Part model, mm, in its own coordinate system. A direction names the side the tool comes from. Give positions to 0.01 mm unless a question says otherwise; leave off trailing zeros. Order: outer loops, then holes, each group sorted by start corner. A loop starts at its lowest first (then second) coordinate and runs counter-clockwise, first axis right, second up.
1. Drop flat-ended pins along their axis: pin 1 Ø0.8 at (y, z) = (3, 2) entering from +X; pin 2 Ø1 at (x, y) = (11, 2) entering from +Z; pin 3 Ø4 at (x, z) = (5, 12.5) entering from -Y; pin 4 Ø1.5 at (x, y) = (5, -4.5) entering from +Z. Give the stop position or say it passes through.
2. Which spindle directions (+Z, -Z, +X, -X, +Y, -Y) get a long thin tool onto all of the face, cutting with end or side? Do faces 1 (the flat face through (14, -1, 3.345)), 2 (the flat face through (14, 1.4, 25)), 3 (the flat face through (22.64, -1, 2)). Say none if no direction does.
3. Mould opens along X. For faces 4 (the flat face through (14, 1, 27.5)), 5 (the flat face through (4.86, -1, 2)), 6 (the flat face through (14, -2.54, 3)), 7 (the cylindrical face through (26.84, 0.69, 1.72)) say: +X half, -X half, draft (parallel to the pull), parting line (faces both ways), or undercut.
4. Probe line 1 (X direction, y = 0.7, z = 1.9); line 2 (Y direction, x = 24.75, z = 16); line 3 (Y direction, x = 17.75, z = 4). List the from-to ranges inside material, lowest first.
5. Slice it at C-C on y = -5.5. List the corners of the cut face in (x, z) (3 decimals), and give its area (3 significant figures).
6. Slice it at B-B on z = 25.6. List the corners of the cut face in (x, y), and give its area (3 significant figures).
7. Slice it at D-D on y = 0.75. List the corners of the cut face in (x, z), and give its area (3 significant figures).
8. Slice it at A-A on x = 2.05. List the corners of the cut face in (y, z), and give its area (3 significant figures).
from build123d import *

# Parameters (mm, degrees)
SKETCH_1_W      = 27.5
SKETCH_1_H      = 27.5
SKETCH_1_R      = 1.4
EXTRUDE_1_DEPTH = 1.4
SKETCH_1_3_W    = 27.5
SKETCH_1_3_H    = 19.2
EXTRUDE_2_DEPTH = 3
SKETCH_1_4_W    = 2.54
SKETCH_1_4_H    = 2.54
EXTRUDE_3_DEPTH = 2.54
EXTRUDE_START   = 3.4
SKETCH_1_5_W    = 0.7
SKETCH_1_5_H    = 0.7
EXTRUDE_4_DEPTH = 11.3


with BuildPart() as part:
    # Sketch 1 → Extrude 1 (new body)
    with BuildSketch(Plane(origin=(0, 0, 0), x_dir=(1, 0, 0), z_dir=(0, 1, 0))):
        with Locations((13.75, -13.75)):
            Rectangle(SKETCH_1_W, SKETCH_1_H)
        with Locations(Location((2.05, -1.9, 0), (0, 0, 270))):
            Circle(SKETCH_1_R, mode=Mode.SUBTRACT)
        with Locations(Location((25.45, -1.9, 0), (0, 0, 270))):
            Circle(SKETCH_1_R, mode=Mode.SUBTRACT)
        with Locations(Location((2.05, -25.6, 0), (0, 0, 270))):
            Circle(SKETCH_1_R, mode=Mode.SUBTRACT)
        with Locations(Location((25.45, -25.6, 0), (0, 0, 270))):
            Circle(SKETCH_1_R, mode=Mode.SUBTRACT)
    extrude(amount=EXTRUDE_1_DEPTH)

    # Sketch 1_3 → Extrude 2 (add)
    with BuildSketch(Plane(origin=(0, 0, 0), x_dir=(1, 0, 0), z_dir=(0, 1, 0))):
        with Locations((13.75, -13.75)):
            Rectangle(SKETCH_1_3_W, SKETCH_1_3_H)
    extrude(amount=EXTRUDE_2_DEPTH)

    # Sketch 1_4 → Extrude 3 (add)
    with BuildSketch(Plane(origin=(0, 0, 0), x_dir=(1, 0, 0), z_dir=(0, 1, 0))):
        with Locations((6.13, -2.075)):
            Rectangle(SKETCH_1_4_W, SKETCH_1_4_H)
        with Locations((8.67, -2.075)):
            Rectangle(SKETCH_1_4_W, SKETCH_1_4_H)
        with Locations((11.21, -2.075)):
            Rectangle(SKETCH_1_4_W, SKETCH_1_4_H)
        with Locations((13.75, -2.075)):
            Rectangle(SKETCH_1_4_W, SKETCH_1_4_H)
        with Locations((16.29, -2.075)):
            Rectangle(SKETCH_1_4_W, SKETCH_1_4_H)
        with Locations((18.83, -2.075)):
            Rectangle(SKETCH_1_4_W, SKETCH_1_4_H)
        with Locations((21.37, -2.075)):
            Rectangle(SKETCH_1_4_W, SKETCH_1_4_H)
    extrude(amount=-EXTRUDE_3_DEPTH)

    # Sketch 1_5 → Extrude 4 (add)
    with BuildSketch(Plane(origin=(0, 0, 0), x_dir=(1, 0, 0), z_dir=(0, 1, 0)).offset(EXTRUDE_START)):
        with Locations((6.13, -2.075)):
            Rectangle(SKETCH_1_5_W, SKETCH_1_5_H)
        with Locations((8.67, -2.075)):
            Rectangle(SKETCH_1_5_W, SKETCH_1_5_H)
        with Locations((11.21, -2.075)):
            Rectangle(SKETCH_1_5_W, SKETCH_1_5_H)
        with Locations((13.75, -2.075)):
            Rectangle(SKETCH_1_5_W, SKETCH_1_5_H)
        with Locations((16.29, -2.075)):
            Rectangle(SKETCH_1_5_W, SKETCH_1_5_H)
        with Locations((18.83, -2.075)):
            Rectangle(SKETCH_1_5_W, SKETCH_1_5_H)
        with Locations((21.37, -2.075)):
            Rectangle(SKETCH_1_5_W, SKETCH_1_5_H)
    extrude(amount=-EXTRUDE_4_DEPTH)


solid = part.part
Data:
1. pin 1: stops at x = 21.72
1. pin 2: stops at z = 23.35
1. pin 3: stops at y = 0
1. pin 4: passes through
2. face 1: +Z, +X, -X, -Y
2. face 2: +Z, +X, -X, +Y
2. face 3: +Z, -Z, +X, -Y
3. face 4: draft
3. face 5: -X half
3. face 6: undercut
3. face 7: undercut
4. line 1: x = 0 to 0.65, 3.45 to 24.05, 26.85 to 27.5
4. line 2: y = 0 to 3
4. line 3: y = 0 to 1.4
5. outline: (5.78, 1.725) - (6.48, 1.725) - (6.48, 2.425) - (5.78, 2.425) - close; (8.32, 1.725) - (9.02, 1.725) - (9.02, 2.425) - (8.32, 2.425) - close; (10.86, 1.725) - (11.56, 1.725) - (11.56, 2.425) - (10.86, 2.425) - close; (13.4, 1.725) - (14.1, 1.725) - (14.1, 2.425) - (13.4, 2.425) - close; (15.94, 1.725) - (16.64, 1.725) - (16.64, 2.425) - (15.94, 2.425) - close; (18.48, 1.725) - (19.18, 1.725) - (19.18, 2.425) - (18.48, 2.425) - close; (21.02, 1.725) - (21.72, 1.725) - (21.72, 2.425) - (21.02, 2.425) - close
5. area: 3.43 mm2
6. outline: (0, 0) - (0.65, 0) - (0.65, 1.4) - (0, 1.4) - close; (3.45, 0) - (24.05, 0) - (24.05, 1.4) - (3.45, 1.4) - close; (26.85, 0) - (27.5, 0) - (27.5, 1.4) - (26.85, 1.4) - close
6. area: 30.7 mm2
7. outline: (0, 0) - (27.5, 0) - (27.5, 27.5) - (0, 27.5) - close; hole circle Ø2.8 at (2.05, 1.9); hole circle Ø2.8 at (2.05, 25.6); hole circle Ø2.8 at (25.45, 1.9); hole circle Ø2.8 at (25.45, 25.6)
7. area: 732 mm2
8. outline: (0, 0) - (1.4, 0) - (1.4, 0.5) - (0, 0.5) - close; (0, 3.3) - (1.4, 3.3) - (1.4, 4.15) - (3, 4.15) - (3, 23.35) - (1.4, 23.35) - (1.4, 24.2) - (0, 24.2) - close; (0, 27) - (1.4, 27) - (1.4, 27.5) - (0, 27.5) - close
8. area: 61.4 mm2
